The listing builds one solid part. Answer for the finished solid, in the listing's coordinates (mm). Round coordinates to 2 decimals unless told otherwise and drop trailing zeros. Write each loop counter-clockwise with the first axis right and the second up, starting at its lowest first coordinate (ties: lowest second). Pieces come first, ordered by that corner, then holes.
Item 1: Find section D-D on z = 29. Give the vertices of the cut face in (x, y), then the cut area to 3 significant figures.
Item 2: Find section B-B on y = 1.1. Give the vertices of the cut face in (x, z), then the cut area to 3 significant figures.
Item 3: Find section A-A on z = 5.5. Give the vertices of the cut face in (x, y).
Item 4: Find the intervals of material crossed by probe 1 along X at (y, z) = (1.2, 52.5); probe 2 along X at (y, z) = (1.05, 53.5); probe 3 along Z at (x, y) = (-4.5, 0.6), in increasing order.
Item 5: This flat-tipped pin is pushed along its axis until it touches: pin 1 (3 mm diameter, centred on x = -4, z = 5.5, fed in from -Y). Where does it stop, or does it pass through?
Item 6: Find section C-C on x = 124. Give the vertices of the cut face in (y, z), then the cut area to 3 significant figures.
```python
from build123d import *

# Parameters (mm, degrees)
SKETCH1_W              = 121
SKETCH1_H              = 58
BOSS_EXTRUDE1_DEPTH    = 3
SKETCH2_W              = 3
SKETCH2_H              = 58
BOSS_EXTRUDE2_DEPTH    = 29
SKETCH3_R              = 2.5
CUT_EXTRUDE1_DEPTH     = 29
CUT_EXTRUDE2_START     = -29
SKETCH4_R              = 2.5
CUT_EXTRUDE2_DEPTH     = 29
CONVERT_SOLID1_DEPTH   = 58
CONVERT_SOLID1_2_DEPTH = 58
UNFOLD1_START          = 3
UNFOLD1_OUTLINE_W      = 121
UNFOLD1_OUTLINE_H      = 58
UNFOLD1_DEPTH          = 29
UNFOLD1_2_OUTLINE_R    = 2.5
UNFOLD1_2_DEPTH        = 3


# Read off the part's stored shape, not the designer's step: Convert-Solid1, Unfold1
with BuildPart() as part:
    # Sketch1 → Boss-Extrude1 (new body)
    with BuildSketch(Plane(origin=(0, 0, 0), x_dir=(1, 0, 0), z_dir=(0, 1, 0))):
        with Locations((60.5, -29)):
            Rectangle(SKETCH1_W, SKETCH1_H)
    extrude(amount=BOSS_EXTRUDE1_DEPTH)

    # Sketch2 → Boss-Extrude2 (add)
    with BuildSketch(Plane(origin=(0, 3, 0), x_dir=(1, 0, 0), z_dir=(0, 1, 0))):
        with Locations((1.5, -29)):
            Rectangle(SKETCH2_W, SKETCH2_H)
        with Locations((119.5, -29)):
            Rectangle(SKETCH2_W, SKETCH2_H)
    extrude(amount=BOSS_EXTRUDE2_DEPTH)

    # Sketch3 → Cut-Extrude1 (cut)
    with BuildSketch(Plane.ZY):
        with Locations((5.5, 8.5)):
            Circle(SKETCH3_R)
        with Locations((52.5, 8.5)):
            Circle(SKETCH3_R)
        with BuildLine():
            Line((9, 32), (49, 32))
            ThreePointArc((49, 32), (29, 12), (9, 32))
        make_face()
    extrude(amount=-CUT_EXTRUDE1_DEPTH, mode=Mode.SUBTRACT)

    # Sketch4 → Cut-Extrude2 (cut)
    with BuildSketch(Plane(origin=(121, 0, 0), x_dir=(0, 0, -1), z_dir=(1, 0, 0)).offset(CUT_EXTRUDE2_START)):
        with Locations(Location((-52.5, 8.5, 0), (0, 0, 180))):
            Circle(SKETCH4_R)
        with Locations(Location((-5.5, 8.5, 0), (0, 0, 180))):
            Circle(SKETCH4_R)
    extrude(amount=CUT_EXTRUDE2_DEPTH, mode=Mode.SUBTRACT)

    # Convert-Solid1 outline → Convert-Solid1 (cut)
    with BuildSketch(Plane.XY):
        with BuildLine():
            Line((0, 0), (5, 0))
            ThreePointArc((5, 0), (1.464466094, 1.464466094), (0, 5))
            Line((0, 5), (0, 0))
        make_face()
        with BuildLine():
            ThreePointArc((121, 5), (119.535533906, 1.464466094), (116, 0))
            Line((116, 0), (121, 0))
            Line((121, 0), (121, 5))
        make_face()
    extrude(amount=CONVERT_SOLID1_DEPTH, mode=Mode.SUBTRACT)

    # Convert-Solid1 2 outline → Convert-Solid1 2 (add)
    with BuildSketch(Plane.XY):
        with BuildLine():
            Line((3, 3), (5, 3))
            ThreePointArc((5, 3), (3.585786438, 3.585786438), (3, 5))
            Line((3, 5), (3, 3))
        make_face()
        with BuildLine():
            ThreePointArc((118, 5), (117.414213562, 3.585786438), (116, 3))
            Line((116, 3), (118, 3))
            Line((118, 3), (118, 5))
        make_face()
    extrude(amount=CONVERT_SOLID1_2_DEPTH)

    # Unfold1 outline → Unfold1 (cut)
    with BuildSketch(Plane(origin=(0, 0, 0), x_dir=(1, 0, 0), z_dir=(0, 1, 0)).offset(UNFOLD1_START)):
        with Locations((60.5, -29)):
            Rectangle(UNFOLD1_OUTLINE_W, UNFOLD1_OUTLINE_H)
    extrude(amount=UNFOLD1_DEPTH, mode=Mode.SUBTRACT)

    # Unfold1 2 outline → Unfold1 2 (add)
    with BuildSketch(Plane(origin=(0, 0, 0), x_dir=(1, 0, 0), z_dir=(0, 1, 0))):
        with BuildLine():
            Line((-27.497787144, 0), (-27.497787144, -9))
            ThreePointArc((-27.497787144, -9), (-7.497787144, -29), (-27.497787144, -49))
            Line((-27.497787144, -49), (-27.497787144, -58))
            Line((-27.497787144, -58), (148.497787144, -58))
            Line((148.497787144, -58), (148.497787144, 0))
            Line((148.497787144, 0), (-27.497787144, 0))
        make_face()
        with Locations((124.997787144, -5.5)):
            Circle(UNFOLD1_2_OUTLINE_R, mode=Mode.SUBTRACT)
        with Locations((124.997787144, -52.5)):
            Circle(UNFOLD1_2_OUTLINE_R, mode=Mode.SUBTRACT)
        with Locations((-3.997787144, -5.5)):
            Circle(UNFOLD1_2_OUTLINE_R, mode=Mode.SUBTRACT)
        with Locations((-3.997787144, -52.5)):
            Circle(UNFOLD1_2_OUTLINE_R, mode=Mode.SUBTRACT)
    extrude(amount=UNFOLD1_2_DEPTH)


solid = part.part
```
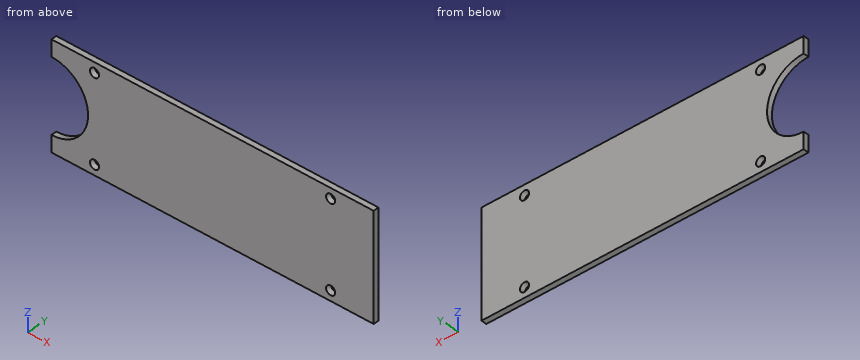
Check values:
1. outline: (-7.5, 0) - (148.5, 0) - (148.5, 3) - (-7.5, 3) - close
1. area: 468 mm2
2. outline: (-27.5, 0) - (148.5, 0) - (148.5, 58) - (-27.5, 58) - (-27.5, 49) arc R20 cw to (-27.5, 9) - close; hole circle Ø5 at (-4, 5.5); hole circle Ø5 at (-4, 52.5); hole circle Ø5 at (125, 5.5); hole circle Ø5 at (125, 52.5)
2. area: 9,500 mm2
3. outline: (-27.5, 0) - (-6.5, 0) - (-6.5, 3) - (-27.5, 3) - close; (-1.5, 0) - (122.5, 0) - (122.5, 3) - (-1.5, 3) - close; (127.5, 0) - (148.5, 0) - (148.5, 3) - (127.5, 3) - close
4. probe 1: x = -27.5 to -6.5, -1.5 to 122.5, 127.5 to 148.5
4. probe 2: x = -27.5 to -6.29, -1.71 to 122.71, 127.29 to 148.5
4. probe 3: z = 0 to 3.05, 7.95 to 50.05, 54.95 to 58
5. pin 1: passes through
6. outline: (0, 0) - (3, 0) - (3, 3.21) - (0, 3.21) - close; (0, 7.79) - (3, 7.79) - (3, 50.21) - (0, 50.21) - close; (0, 54.79) - (3, 54.79) - (3, 58) - (0, 58) - close
6. area: 146 mm2
